```python
from build123d import *

# Parameters (mm, degrees)
F0_R     = 5
F1_DEPTH = 60
F2_R     = 5
F3_DEPTH = 30
F4_R     = 1


with BuildPart() as f1:
    # F0 (on Front) → F1 (new body, symmetric)
    with BuildSketch(Plane.XZ):
        Circle(F0_R)
    extrude(amount=F1_DEPTH, both=True)

    # F2 (on Top) → F3 (join)
    with BuildSketch(Plane.XY):
        with Locations((0, 48)):
            Circle(F2_R)
        with Locations((0, -48)):
            Circle(F2_R)
    extrude(amount=F3_DEPTH)

    # F4
    f4_edges = [f1.edges().sort_by_distance(p)[0] for p in [
        (-5, 60, 0),
        (-5, -60, 0),
    ]]
    fillet(f4_edges, radius=F4_R)


solid = f1.part
```
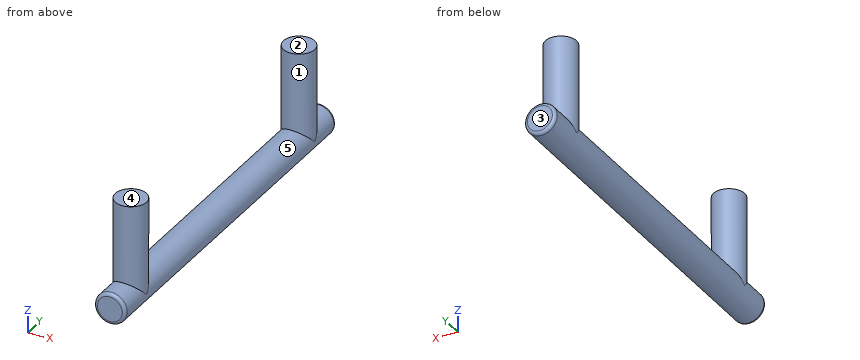
Check sheet for the modelled part. Datum: model origin and axes. Units: mm. Face numbers are marked on the shaded views. A direction names the side the tool comes from. Give positions to 0.01 mm unless a question says otherwise; leave off trailing zeros. Write each loop counter-clockwise with the first axis right and the second up, starting at its lowest first coordinate (ties: lowest second). Pieces come first, ordered by that corner, then holes. Notation, with made-up numbers: (-37, 51) - (9, 51) arc R21 ccw to (9, 88) - close; hole circle Ø1 at (-13.75, 58.25). An arc over 180 degrees is marked (long way). Answer as a JSON object with one key per item and string values. Group by question number.
1) Depth check by flat-ended pin: P1, Ø6, axis at x = 4, z = 8.5, coming from the +Y side; P2, Ø6, axis at x = -1, y = -20, coming from the +Z side; P3, Ø6, axis at x = 1.5, z = 20.5, coming from the +Y side. Enter the tip coordinate at first touch or a pass-through.
2) Sectioned sample at D-D (y = -38). Record the cut outline in (x, z).
3) Sectioned sample at B-B (z = 21.5). Record the cut outline in (x, y), then the cut area to 3 significant figures.
4) Sectioned sample at C-C (y = 48). Record the cut outline in (x, z), then the cut area to 3 significant figures.
5) Sectioned sample at A-A (x = 0). Record the cut outline in (y, z).
6) Access from +Z, -Z, +X, -X, +Y, -Y to the whole of each face (thin tool, end or side, straight path). Record for the marked faces 1 and 2.
7) Thickness scan on probe 1 along Y at (x, z) = (0.5, 25); probe 2 along Z at (x, y) = (-0.25, -20); probe 3 along Y at (x, z) = (-4, 23). Record the ranges inside material, lowest first. Write a range as from..to.
8) Release check for a two-part mould opening along Y. For the marked faces 3, 4 and 5 record: pulls with the +Y half, pulls with the -Y half, needs draft (parallel to the pull), parting line crosses it, or undercut.
Geometry results:
{
 "1": {"P1": "stops at y = 52.9", "P2": "stops at z = 5", "P3": "stops at y = 53"},
 "2": {"outline": "circle Ø10 at (0, 0)"},
 "3": {"outline": "circle Ø10 at (0, -48); circle Ø10 at (0, 48)", "area": "157 mm^2"},
 "4": {"outline": "(-5, 0) arc R5 ccw to (5, 0) - (5, 30) - (-5, 30) - close", "area": "339 mm^2"},
 "5": {"outline": "(-60, -4) arc R1 ccw to (-59, -5) - (59, -5) arc R1 ccw to (60, -4) - (60, 4) arc R1 ccw to (59, 5) - (53, 5) - (53, 30) - (43, 30) - (43, 5) - (-43, 5) - (-43, 30) - (-53, 30) - (-53, 5) - (-59, 5) arc R1 ccw to (-60, 4) - close"},
 "6": {"face 1": "+Z", "face 2": "+Z, +X, -X, +Y, -Y"},
 "7": {"probe 1": "y = -52.97..-43.03, 43.03..52.97", "probe 2": "z = -4.99..4.99", "probe 3": "y = -51..-45, 45..51"},
 "8": {"face 3": "pulls with the +Y half", "face 4": "needs draft", "face 5": "undercut"}
}
